Autodesk Inventor part; units mm, degrees
ref_plane "Plano inicial" through (0, 0, 50) normal (0, 0, 1) x (1, 0, 0)
ref_plane "Plano final" through (0, 0, 502.5) normal (0, 0, 1) x (1, 0, 0)
ref_plane "Plano de trabajo4" through (-11.25, -155, 502.5) normal (0, 0, 1) x (1, 0, 0)
ref_plane "Plano inicial" through (0, 0, 50) normal (0, 0, 1) x (1, 0, 0)
ref_plane "Plano final" through (0, 0, 502.5) normal (0, 0, 1) x (1, 0, 0)
sketch "Boceto" plane through (0, 0, 0) normal (0, 0, 1) x (1, 0, 0)
  line L0 (-10, -16) -> (-10, 16)
  line L1 (-6, 20) -> (6, 20)
  line L2 (10, 16) -> (10, -16)
  line L3 (6, -20) -> (-6, -20)
  arc A0 (-10, -16) -> (-6, -20) centre (-6, -16) ccw
  arc A1 (10, 16) -> (6, 20) centre (6, 16) ccw
  arc A2 (-6, 20) -> (-10, 16) centre (-6, 16) ccw
  arc A3 (6, -20) -> (10, -16) centre (6, -16) ccw
  arc A4 (-6, 18) -> (-8, 16) centre (-6, 16) ccw
  line L4 (-6, 18) -> (6, 18)
  arc A5 (8, 16) -> (6, 18) centre (6, 16) ccw
  line L5 (8, 16) -> (8, -16)
  arc A6 (6, -18) -> (8, -16) centre (6, -16) ccw
  line L6 (6, -18) -> (-6, -18)
  arc A7 (-8, -16) -> (-6, -18) centre (-6, -16) ccw
  line L7 (-8, -16) -> (-8, 16)
  line L8 (0, 29.1598) -> (0, -29.1598) construction
  line L9 (-15.1598, 0) -> (15.1598, 0) construction
  dimension "d7" = 4
  dimension "d9" = 20
  dimension "d11" = 40
  dimension "d12" = 2
  dimension "d15" = 10
  dimension "d16" = 20
extrude "Cuerpo" add sketch "Boceto" along normal up to surface (452.5 mm away) from surface at 50
sketch "Sketch3" plane through (0, 0, 0) normal (0, 0, 1) x (1, 0, 0)
  line L0 (0, 0) -> (10, 0)
ref_plane "Work Plane3" through (0, 0, 0) normal (0, -1, 0) x (1, 0, 0)
sketch "Sketch4" plane through (0, 0, 0) normal (0, -1, 0) x (1, 0, 0)
  line L0 (-2, 50) -> (12, 50)
  line L1 (-2, 502.5) -> (12, 502.5)
  dimension "d18" = 452.5
ref_plane "Plano de trabajo4" through (-11.25, -155, 502.5) normal (0, 0, 1) x (1, 0, 0)
split "Dividir1" plane through (-11.25, -155, 502.5) removes the side toward (0, 0, 1)
ref_plane "Plano de trabajo5" through (6.25, 20, 50) normal (0, 0, -1) x (-1, 0, 0)
split "Dividir2" plane through (6.25, 20, 50) removes the side toward (0, 0, -1)
equation "\"d7\" = G_IR"
equation "\"d9\" = G_W"
equation "\"d11\" = G_H"
equation "\"d12\" = G_T"
equation "\"d15\" = 0.5 * d9"
equation "\"d16\" = 0.5 * d11"
equation "\"d3\" = G_L"
equation "\"G_W\" = 20"
equation "\"G_H\" = 40"
equation "\"G_T\" = 2"
equation "\"G_IR\" = 4"
equation "\"G_L\" = d18"
equation "\"G_OFFSET_END\" = -47.5"
equation "\"d14\" = G_OFFSET_END + B_L"
properties part number "ISO 4019 - 40x20x2 - 452,5" material "Acero, suave"
Verification items for the finished model (mm, model axes). A direction names the side the tool comes from. Give positions to 0.01 mm unless a question says otherwise; leave off trailing zeros. Order: outer loops, then holes, each group sorted by start corner. A loop starts at its lowest first (then second) coordinate and runs counter-clockwise, first axis right, second up. Notation, with made-up numbers: M 84.25,6 L 128.25,6 A27 cw 128.25,36 Z; hole C 85,71 d7. An arc over 180 degrees is marked long. Use one line per item in the form item = value. Start each with the question number.
Q1. Scan lines: line 1 along X through (y, z) = (-15.5, 282.5); line 2 along Y through (x, z) = (4.5, 264.5); line 3 along Y through (x, z) = (7.75, 407). Record each from-to range of solid material in increasing order. Write a range as [from, to].
Q2. Access from +Z, -Z, +X, -X, +Y, -Y to the whole of each face (thin tool, end or side, straight path). Record for faces 1 (the flat face through (0, 18, 273)), 2 (the flat face through (-8.2, 0.1, 50)).
Q3. Section check A-A (y = 12). Enter the section's corners in (x, z).
Q4. Section check C-C (x = 2.5). Enter the section's corners in (y, z).
Q5. Mould release check, pull along Y, two halves, no side actions. Record for faces 3 (the flat face through (0, 20, 273)), 4 (the flat face through (-8.2, 0.1, 502.5)), 5 (the flat face through (0, -20, 273)), 6 (the flat face through (8, 0, 273)): +Y half, -Y half, draft (parallel to the pull), parting line (faces both ways), or undercut.
Q6. Section check B-B (z = 99). Enter the section's corners in (x, y).
Evaluation:
q1.line_1 = [-10, -8], [8, 10]
q1.line_2 = [-20, -18], [18, 20]
q1.line_3 = [-19.6, -16.97], [16.97, 19.6]
q2.face_1 = +Z, -Z
q2.face_2 = -Z, +X, -X, +Y, -Y
q3.outline = M -10,50 L -8,50 L -8,502.5 L -10,502.5 Z; M 8,50 L 10,50 L 10,502.5 L 8,502.5 Z
q4.outline = M -20,50 L -18,50 L -18,502.5 L -20,502.5 Z; M 18,50 L 20,50 L 20,502.5 L 18,502.5 Z
q5.face_3 = +Y half
q5.face_4 = draft
q5.face_5 = -Y half
q5.face_6 = undercut
q6.outline = M -10,-16 A4 ccw -6,-20 L 6,-20 A4 ccw 10,-16 L 10,16 A4 ccw 6,20 L -6,20 A4 ccw -10,16 Z; hole M -8,-16 A2 ccw -6,-18 L 6,-18 A2 ccw 8,-16 L 8,16 A2 ccw 6,18 L -6,18 A2 ccw -8,16 Z
